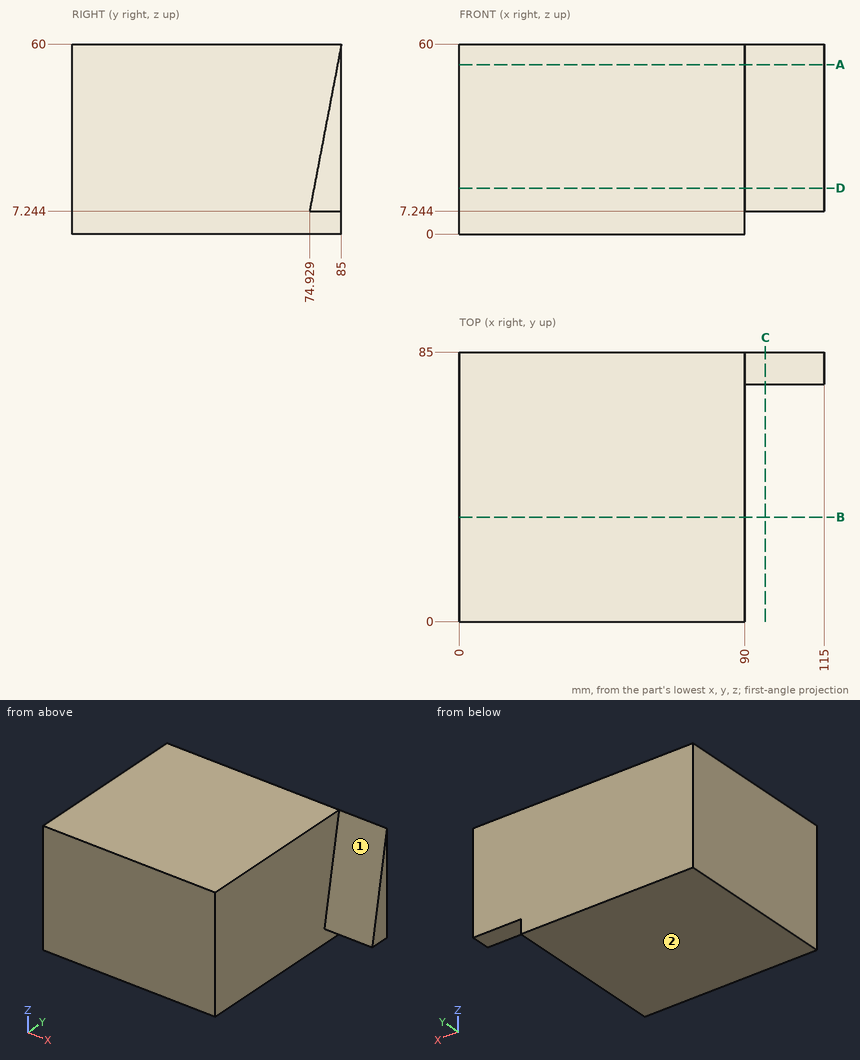
Print and shaded views of the part. All mm, measured from the part's lowest x, y and z. A direction names the side the tool comes from. Coordinates: 2 decimals unless noted, no trailing zeros. Order: outer loops, then holes, each group sorted by start corner. A loop starts at its lowest first (then second) coordinate and runs counter-clockwise, first axis right, second up.
Item 1: Saw through at B-B on y = 33. List the corners of the cut face in (x, z), then the cut area to 3 significant figures.
Filled in:
outline: (0, 0) - (90, 0) - (90, 60) - (0, 60) - close
area: 5,400 mm2
Item 2: Saw through at C-C on x = 96.5. List the corners of the cut face in (y, z).
Filled in:
outline: (74.93, 7.24) - (85, 7.24) - (85, 60) - close
Item 3: Tool access for the marked faces 1 and 2: list every direction of +Z, -Z, +X, -X, +Y, -Y with a clear straight run to the whole face (end or side of a thin tool).
Filled in:
face 1: +Z, +X, -Y
face 2: -Z, +X, -X, +Y, -Y
Item 4: Drop flat-ended pins along their axis: pin 1 Ø8 at (x, y) = (106, 77.5) entering from -Z; pin 2 Ø8 at (x, z) = (65, 23.5) entering from -Y; pin 3 Ø6 at (y, z) = (26.5, 7) entering from +X; pin 4 Ø1.5 at (x, y) = (92.5, 46) entering from +Z. Give the stop position or say it passes through.
Filled in:
pin 1: stops at z = 7.24
pin 2: stops at y = 0
pin 3: stops at x = 90
pin 4: passes through
Item 5: Drill centre lines: L1, parallel to X at y = 34, z = 16; L2, parallel to Y at x = 95, z = 31 (1 decimal); L3, parallel to Y at x = 104, z = 52. Where is each one in solid material? Low to high.
Filled in:
L1: x = 0 to 90
L2: y = 79.5 to 85
L3: y = 83.47 to 85
Item 6: Saw through at A-A on z = 53.5. List the corners of the cut face in (x, y), then the cut area to 3 significant figures.
Filled in:
outline: (0, 0) - (90, 0) - (90, 83.76) - (115, 83.76) - (115, 85) - (0, 85) - close
area: 7,680 mm2
Item 7: Saw through at D-D on z = 14.5. List the corners of the cut face in (x, y) (1 decimal), then the cut area to 3 significant figures.
Filled in:
outline: (0, 0) - (90, 0) - (90, 76.3) - (115, 76.3) - (115, 85) - (0, 85) - close
area: 7,870 mm2
